```python
from build123d import *

# Parameters (mm, degrees)
SKETCH2_W           = 93.2
SKETCH2_H           = 75.1
SKETCH2_R           = 1.7
BOSS_EXTRUDE2_DEPTH = 5
FILLET1_R           = 5
SKETCH4_R           = 3.2
SKETCH4_R_2         = 1.7
BOSS_EXTRUDE3_DEPTH = 7.5
SKETCH6_W           = 10
SKETCH6_H           = 32
CUT_EXTRUDE1_DEPTH  = 6
BOSS_EXTRUDE4_DEPTH = 5


with BuildPart() as part:
    # Sketch2 → Boss-Extrude2 (new body)
    with BuildSketch(Plane(origin=(0, 0, 0), x_dir=(1, 0, 0), z_dir=(0, 1, 0))):
        Rectangle(SKETCH2_W, SKETCH2_H)
        with Locations((-41.6, 32.55)):
            Circle(SKETCH2_R, mode=Mode.SUBTRACT)
        with Locations((41.6, 32.55)):
            Circle(SKETCH2_R, mode=Mode.SUBTRACT)
        with Locations((41.6, -32.55)):
            Circle(SKETCH2_R, mode=Mode.SUBTRACT)
        with Locations((-41.6, -32.55)):
            Circle(SKETCH2_R, mode=Mode.SUBTRACT)
        Polygon((-36.6, -24.420896868), (-36.6, 24.420896868), (-4.156993635, 0), align=None, mode=Mode.SUBTRACT)
        Polygon((36.6, -24.420896868), (36.6, 24.420896868), (4.156993635, 0), align=None, mode=Mode.SUBTRACT)
        Polygon((32.443006365, -27.55), (-32.443006365, -27.55), (0, -3.129103132), align=None, mode=Mode.SUBTRACT)
        Polygon((-32.443006365, 27.55), (0, 3.129103132), (32.443006365, 27.55), align=None, mode=Mode.SUBTRACT)
    extrude(amount=BOSS_EXTRUDE2_DEPTH)

    # Fillet1
    fillet1_edges = [part.edges().sort_by_distance(p)[0] for p in [
        (0, 2.5, 3.129103132),
        (-4.156993635, 2.5, 0),
        (4.156993635, 2.5, 0),
        (0, 2.5, -3.129103132),
    ]]
    fillet(fillet1_edges, radius=FILLET1_R)

    # Sketch4 → Boss-Extrude3 (add)
    with BuildSketch(Plane(origin=(0, 5, 0), x_dir=(1, 0, 0), z_dir=(0, 1, 0))):
        with Locations((-41.6, 32.55)):
            Circle(SKETCH4_R)
        with Locations((-41.6, 32.55)):
            Circle(SKETCH4_R_2, mode=Mode.SUBTRACT)
        with Locations((41.6, 32.55)):
            Circle(SKETCH4_R)
        with Locations((41.6, 32.55)):
            Circle(SKETCH4_R_2, mode=Mode.SUBTRACT)
        with Locations((-41.6, -32.55)):
            Circle(SKETCH4_R)
        with Locations((-41.6, -32.55)):
            Circle(SKETCH4_R_2, mode=Mode.SUBTRACT)
        with Locations((41.6, -32.55)):
            Circle(SKETCH4_R)
        with Locations((41.6, -32.55)):
            Circle(SKETCH4_R_2, mode=Mode.SUBTRACT)
    extrude(amount=BOSS_EXTRUDE3_DEPTH)

    # Sketch6 → Cut-Extrude1 (cut, through all)
    with BuildSketch(Plane(origin=(0, 5, 0), x_dir=(1, 0, 0), z_dir=(0, 1, 0))):
        with Locations((-41.6, 0)):
            Rectangle(SKETCH6_W, SKETCH6_H)
    extrude(amount=-CUT_EXTRUDE1_DEPTH, mode=Mode.SUBTRACT)

    # Sketch7 → Boss-Extrude4 (add)
    with BuildSketch(Plane(origin=(0, 5, 0), x_dir=(1, 0, 0), z_dir=(0, 1, 0))):
        Polygon((-36.6, 16), (-34.6, 16), (-34.6, -16), (-36.6, -16), (-36.6, -24.420896868), (-29.6, -19.151771185), (-29.6, 19.151771185), (-36.6, 24.420896868), align=None)
    extrude(amount=-BOSS_EXTRUDE4_DEPTH)


solid = part.part
```
Could you check a few things on this model? Use its own coordinates, in mm. A direction names the side the tool comes from. Give positions to 0.01 mm unless a question says otherwise; leave off trailing zeros. Loops run counter-clockwise (first coordinate to the right, second up) from the corner with the lowest first, then second, coordinate; pieces in that order, holes last. Notation, with made-up numbers: (37.25, 12.25) - (92.25, 12.25) arc R18 ccw to (92.25, 36.25) - close; hole circle Ø1 at (50.25, 85.25). An arc over 180 degrees is marked (long way). Answer in a Markdown table with one row per item. Add a question column.
Q1. For pin 1 (1.5 mm diameter, centred on y = 2.5, z = -1.5, fed in from -X); pin 2 (3 mm diameter, centred on x = 28.5, y = 7, fed in from -Z); pin 3 (5.5 mm diameter, centred on x = -41.6, z = -32.55, fed in from +Y); pin 4 (8 mm diameter, centred on x = -30, z = -15.5, fed in from +Y), each with a flat end and sliding along its axis, tell me the tip position at first contact or that it passes through.
Q2. If we section it at B-B (x = 41.6): List the corners of the cut face in (y, z) for me.
Q3. If we section it at C-C (y = 2.25): State how many separate pieces and enclosed holes the cut face has, plus the area to 3 significant figures.
Q4. Which directions (+Z, -Z, +X, -X, +Y, -Y) give clear straight access to the entire face, cutting with the end or side of a thin tool? Please do faces 4 (the face through (-1, 0, -1)), 5 (the face through (-38.644, 8.698, 33.776)), 6 (the face through (-17.931, 2.465, 16.626)).
Q5. We'd pull the mould along Z, two halves only. Please class faces 1 (the face through (-1, 5, -1)), 2 (the face through (-1, 2, -37.55)), 3 (the face through (46.6, 2, 1)): +Z half, -Z half, draft (parallel to the pull), parting line (faces both ways), or undercut.
Q6. Please list where these lines run through material, in increasing order: L1, parallel to Z at x = 41.6, y = 8; L2, parallel to X at y = 8.75, z = -32.55; L3, parallel to Z at x = 41.6, y = 4. Write a range as from..to.
Q7. If we section it at A-A (y = 6.5): List the corners of the cut face in (x, z) for me, plus the area to 3 significant figures.
Q8. If we section it at D-D (x = -41.6): List the corners of the cut face in (y, z) for me, plus the area to 4 significant figures.
The answers:
| question | item | result |
|---|---|---|
| 1 | pin 1 | stops at x = -34.6 |
| 1 | pin 2 | passes through |
| 1 | pin 3 | stops at y = 12.5 |
| 1 | pin 4 | stops at y = 5 |
| 2 | outline | (0, -37.55) - (5, -37.55) - (5, -35.75) - (12.5, -35.75) - (12.5, -34.25) - (0, -34.25) - close; (0, -30.85) - (12.5, -30.85) - (12.5, -29.35) - (5, -29.35) - (5, 29.35) - (12.5, 29.35) - (12.5, 30.85) - (0, 30.85) - close; (0, 34.25) - (12.5, 34.25) - (12.5, 35.75) - (5, 35.75) - (5, 37.55) - (0, 37.55) - close |
| 3 | separate pieces | 1 |
| 3 | enclosed holes | 8 |
| 3 | area | 3,740 mm^2 |
| 4 | face 4 | +Z, -Z, +X, -X, -Y |
| 4 | face 5 | +Y |
| 4 | face 6 | +Y, -Y |
| 5 | face 1 | undercut |
| 5 | face 2 | -Z half |
| 5 | face 3 | draft |
| 6 | L1 | z = -35.75..-34.25, -30.85..-29.35, 29.35..30.85, 34.25..35.75 |
| 6 | L2 | x = -44.8..-43.3, -39.9..-38.4, 38.4..39.9, 43.3..44.8 |
| 6 | L3 | z = -37.55..-34.25, -30.85..30.85, 34.25..37.55 |
| 7 | outline | circle Ø6.4 at (-41.6, -32.55); circle Ø6.4 at (-41.6, 32.55); circle Ø6.4 at (41.6, -32.55); circle Ø6.4 at (41.6, 32.55); hole circle Ø3.4 at (-41.6, -32.55); hole circle Ø3.4 at (-41.6, 32.55); hole circle Ø3.4 at (41.6, -32.55); hole circle Ø3.4 at (41.6, 32.55) |
| 7 | area | 92.4 mm^2 |
| 8 | outline | (0, -37.55) - (5, -37.55) - (5, -35.75) - (12.5, -35.75) - (12.5, -34.25) - (0, -34.25) - close; (0, -30.85) - (12.5, -30.85) - (12.5, -29.35) - (5, -29.35) - (5, -16) - (0, -16) - close; (0, 16) - (5, 16) - (5, 29.35) - (12.5, 29.35) - (12.5, 30.85) - (0, 30.85) - close; (0, 34.25) - (12.5, 34.25) - (12.5, 35.75) - (5, 35.75) - (5, 37.55) - (0, 37.55) - close |
| 8 | area | 226.5 mm^2 |
